For this review, take the finished solid that the model builds, in its own axes (mm). Face numbers are marked on the shaded views. Round coordinates to 2 decimals unless told otherwise and drop trailing zeros. Loops run counter-clockwise (first coordinate to the right, second up) from the corner with the lowest first, then second, coordinate; pieces in that order, holes last. Notation, with made-up numbers: M 39,-22 L 60,-22 A16 ccw 60,-15 Z; hole C 44.25,-23.75 d9. An arc over 180 degrees is marked long. Write item = value, one per line. Start each with the question number.
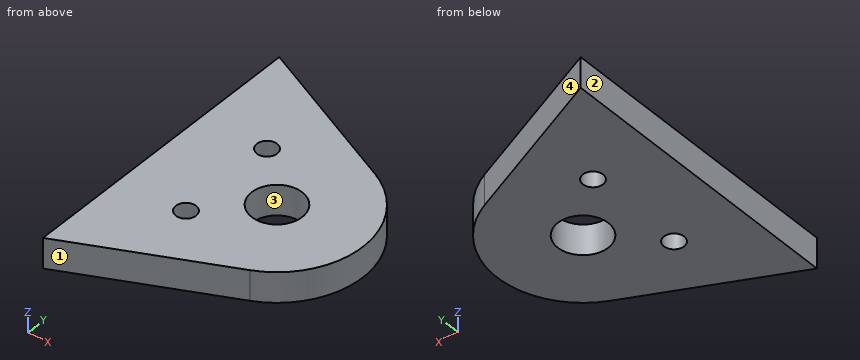
```python
from build123d import *

# Parameters (mm, degrees)
ESQUISSE1_R                  = 19.25
ESQUISSE1_R_2                = 2.5
BOSS_EXTRU_1_DEPTH           = 42
ENL_V_MAT_EXTRU_1_DEPTH      = 74.881298321
ENL_V_MAT_EXTRU_1_DEPTH_BACK = 74.881298321
ESQUISSE2_W                  = 90
ESQUISSE2_H                  = 30
ESQUISSE3_R                  = 1
ENL_V_MAT_EXTRU_2_DEPTH      = 42
ENL_V_MAT_EXTRU_3_DEPTH      = 78.729096869
ENL_V_MAT_EXTRU_3_DEPTH_BACK = 78.729096869
ESQUISSE4_W                  = 87.75
ESQUISSE4_H                  = 33
ESQUISSE4_H_2                = 6


with BuildPart() as part:
    # Esquisse1 → Boss.-Extru.1 (new body)
    with BuildSketch(Plane.XY):
        with BuildLine():
            Line((12.13875, 26.612276273), (53.5275, 7.733481994))
            ThreePointArc((53.5275, 7.733481994), (58.5, 0), (53.5275, -7.733481994))
            Line((53.5275, -7.733481994), (12.13875, -26.612276273))
            ThreePointArc((12.13875, -26.612276273), (-29.25, 0), (12.13875, 26.612276273))
        make_face()
        with Locations(Location((0, 0, 0), (0, 0, 180))):
            Circle(ESQUISSE1_R, mode=Mode.SUBTRACT)
        with Locations(Location((50, 0, 0), (0, 0, 180))):
            Circle(ESQUISSE1_R_2, mode=Mode.SUBTRACT)
    extrude(amount=BOSS_EXTRU_1_DEPTH)

    # Esquisse2 → Enlèv. mat.-Extru.1 (cut, two sides: drawn at the far end of the back side and taken through both)
    with BuildSketch(Plane(origin=(5.218823759, 0, 0), x_dir=(1, 0, 0), z_dir=(0, 1, 0)).offset(-ENL_V_MAT_EXTRU_1_DEPTH_BACK)):
        with Locations((-11.691323759, -21)):
            Rectangle(ESQUISSE2_W, ESQUISSE2_H)
    extrude(amount=ENL_V_MAT_EXTRU_1_DEPTH + ENL_V_MAT_EXTRU_1_DEPTH_BACK, mode=Mode.SUBTRACT)

    # Esquisse3 → Enlèv. mat.-Extru.2 (cut)
    with BuildSketch(Plane.XY.offset(42)):
        with Locations((45, 5)):
            Circle(ESQUISSE3_R)
        with Locations((45, -5)):
            Circle(ESQUISSE3_R)
        with Locations((-15, 19)):
            Circle(ESQUISSE3_R)
        with Locations((-15, -19)):
            Circle(ESQUISSE3_R)
    extrude(amount=-ENL_V_MAT_EXTRU_2_DEPTH, mode=Mode.SUBTRACT)

    # Esquisse4 → Enlèv. mat.-Extru.3 (cut, two sides: drawn at the far end of the back side and taken through both)
    with BuildSketch(Plane(origin=(0, 0, 0), x_dir=(1, 0, 0), z_dir=(0, 1, 0)).offset(-ENL_V_MAT_EXTRU_3_DEPTH_BACK)):
        with Locations((14.625, -25.5)):
            Rectangle(ESQUISSE4_W, ESQUISSE4_H)
        with Locations((14.625, -3)):
            Rectangle(ESQUISSE4_W, ESQUISSE4_H_2)
    extrude(amount=ENL_V_MAT_EXTRU_3_DEPTH + ENL_V_MAT_EXTRU_3_DEPTH_BACK, mode=Mode.SUBTRACT)


solid = part.part
```
(1) Add section C-C on x = 45. Write out the cut boundary in (y, z), and give its area (3 significant figures).
(2) For pin 1 Ø2.5 at (x, y) = (45, 5) entering from -Z, flat-tipped, find the tip position at first contact; note if it passes through.
(3) Add section D-D on y = 5. Write out the cut boundary in (x, z), and give its area (3 significant figures).
(4) Wall thickness on L1, parallel to Y at x = 45, z = 6.9; L2, parallel to Y at x = 44.25, z = 7.65; L3, parallel to Y at x = 50, z = 6.9: over which ranges is each line inside the solid? List them lowest first.
(5) Draft analysis for pull direction Y (two halves, no side actions). For the marked faces 1, 2, 3 and 4, state which applies: +Y half, -Y half, draft (parallel to the pull), parting line (faces both ways), or undercut.
(6) Add section B-B on z = 6.4. Write out the cut boundary in (x, y).
(7) Add section A-A on y = 0. Write out the cut boundary in (x, z).
Answer sheet:
q1.outline = M -11.62,6 L -6,6 L -6,9 L -11.62,9 Z; M -4,6 L 4,6 L 4,9 L -4,9 Z; M 6,6 L 11.62,6 L 11.62,9 L 6,9 Z
q1.area = 57.7 mm²
q2.pin_1 = 6
q3.outline = M 38.53,6 L 44,6 L 44,9 L 38.53,9 Z; M 46,6 L 56.87,6 L 56.87,9 L 46,9 Z
q3.area = 49.0 mm²
q4.L1 = -11.62 to -6, -4 to 4, 6 to 11.62
q4.L2 = -11.97 to -5.66, -4.34 to 4.34, 5.66 to 11.97
q4.L3 = -9.34 to -2.5, 2.5 to 9.34
q5.face_1 = -Y half
q5.face_2 = draft
q5.face_3 = undercut
q5.face_4 = +Y half
q6.outline = M 38.53,-14.58 L 53.53,-7.73 A8.5 ccw 53.53,7.73 L 38.53,14.58 Z; hole C 45,-5 d2; hole C 45,5 d2; hole C 50,0 d5
q7.outline = M 38.53,6 L 47.5,6 L 47.5,9 L 38.53,9 Z; M 52.5,6 L 58.5,6 L 58.5,9 L 52.5,9 Z
